Check sheet for the modelled part. Datum: model origin and axes. Units: mm. Coordinates: 2 decimals unless noted, no trailing zeros. Loops run counter-clockwise (first coordinate to the right, second up) from the corner with the lowest first, then second, coordinate; pieces in that order, holes last.
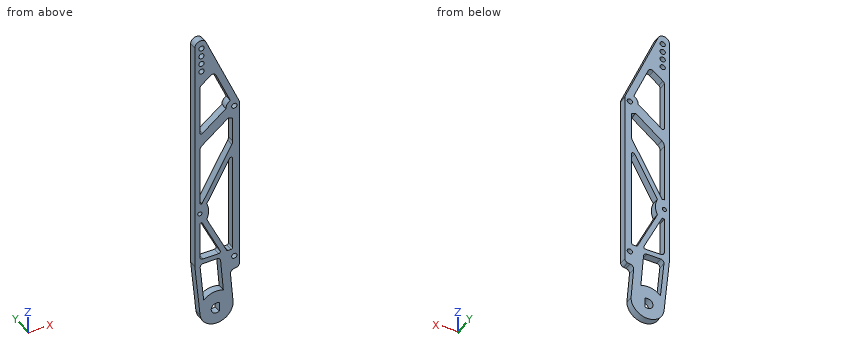
from build123d import *

# Parameters (mm, degrees)
SKETCH2_R           = 2
SKETCH2_R_2         = 1.5875
SKETCH2_R_3         = 1.999999991
BOSS_EXTRUDE1_DEPTH = 5.588


with BuildPart() as part:
    # Sketch2 → Boss-Extrude1 (new body)
    with BuildSketch(Plane(origin=(0, 0, 0), x_dir=(1, 0, 0), z_dir=(0, 1, 0))):
        with BuildLine():
            ThreePointArc((17.295902343, -30.526810701), (16.688093876, -28.878103365), (15.15555913, -28.018449791))
            Line((15.15555913, -28.018449791), (13.238676936, -27.713033224))
            ThreePointArc((13.238676936, -27.713033224), (11.241051513, -26.538356195), (10.573787778, -24.319092227))
            Line((10.573787778, -24.319092227), (12.5603, 0))
            ThreePointArc((12.5603, 0), (0.603657177, 12.545785512), (-12.502275592, 1.2059192))
            Line((-12.502275592, 1.2059192), (-16.498266045, -40.222207921))
            ThreePointArc((-16.498266045, -40.222207921), (-16.507064815, -40.344000039), (-16.51, -40.466074291))
            Line((-16.51, -40.466074291), (-16.51, -221.328861788))
            ThreePointArc((-16.51, -221.328861788), (-12.970187584, -225.680718913), (-7.988667969, -223.101301399))
            Line((-7.988667969, -223.101301399), (16.979901226, -165.677523619))
            ThreePointArc((16.979901226, -165.677523619), (17.216065593, -164.934164738), (17.295902343, -164.158289667))
            Line((17.295902343, -164.158289667), (17.295902343, -30.526810701))
        make_face()
        with Locations(Location((-11.43, -219.075, 0), (0, 0, 270))):
            Circle(SKETCH2_R, mode=Mode.SUBTRACT)
        with Locations(Location((-11.43, -212.725, 0), (0, 0, 270))):
            Circle(SKETCH2_R, mode=Mode.SUBTRACT)
        with Locations(Location((-11.43, -206.375, 0), (0, 0, 270))):
            Circle(SKETCH2_R, mode=Mode.SUBTRACT)
        with Locations(Location((-11.43, -200.025, 0), (0, 0, 270))):
            Circle(SKETCH2_R, mode=Mode.SUBTRACT)
        with BuildLine():
            ThreePointArc((7.135902343, -162.410770806), (8.023611961, -165.648962244), (10.438542905, -167.981776143))
            Line((10.438542905, -167.981776143), (-0.534170778, -193.217289931))
            ThreePointArc((-0.534170778, -193.217289931), (-2.234040931, -194.665234867), (-4.420389569, -194.211381682))
            Line((-4.420389569, -194.211381682), (-11.716886202, -188.551043102))
            ThreePointArc((-11.716886202, -188.551043102), (-12.441018517, -187.661516081), (-12.7, -186.544128716))
            Line((-12.7, -186.544128716), (-12.7, -149.615408258))
            ThreePointArc((-12.7, -149.615408258), (-11.988693683, -148.474898999), (-10.651556899, -148.611951065))
            Line((-10.651556899, -148.611951065), (7.135902343, -162.410770806))
        make_face(mode=Mode.SUBTRACT)
        with BuildLine():
            ThreePointArc((12.215902343, -152.970817152), (10.520298026, -153.359206519), (8.923603828, -154.049487576))
            Line((8.923603828, -154.049487576), (-10.733772403, -138.80005889))
            ThreePointArc((-10.733772403, -138.80005889), (-12.182037035, -137.021004847), (-12.7, -134.786230117))
            Line((-12.7, -134.786230117), (-12.7, -90.4875))
            ThreePointArc((-12.7, -90.4875), (-11.888769677, -90.445936399), (-11.086035141, -90.321680879))
            Line((-11.086035141, -90.321680879), (11.575760855, -131.079432803))
            ThreePointArc((11.575760855, -131.079432803), (12.053263487, -132.272915946), (12.215902343, -133.548047069))
            Line((12.215902343, -133.548047069), (12.215902343, -152.970817152))
        make_face(mode=Mode.SUBTRACT)
        with Locations(Location((13.485902343, -162.410770806, 0), (0, 0, 270))):
            Circle(SKETCH2_R, mode=Mode.SUBTRACT)
        with Locations(Location((-12.7, -82.55, 0), (0, 0, 270))):
            Circle(SKETCH2_R_2, mode=Mode.SUBTRACT)
        with BuildLine():
            Line((-10.16, -44.337182032), (1.663048834, -44.337182032))
            ThreePointArc((1.663048834, -44.337182032), (2.739129831, -44.932682449), (2.806066447, -46.160725831))
            Line((2.806066447, -46.160725831), (-11.055993219, -74.784618621))
            ThreePointArc((-11.055993219, -74.784618621), (-11.873503915, -74.655646925), (-12.7, -74.6125))
            Line((-12.7, -74.6125), (-12.7, -46.877182032))
            ThreePointArc((-12.7, -46.877182032), (-11.956051224, -45.081130808), (-10.16, -44.337182032))
        make_face(mode=Mode.SUBTRACT)
        with BuildLine():
            ThreePointArc((-9.903213406, -40.527182032), (-11.783508673, -39.694838236), (-12.431479451, -37.743315662))
            Line((-12.431479451, -37.743315662), (-9.755434212, -9.99962016))
            ThreePointArc((-9.755434212, -9.99962016), (-2.756273581, -13.695395429), (5.127655889, -12.99492382))
            Line((5.127655889, -12.99492382), (3.069264048, -38.19397392))
            ThreePointArc((3.069264048, -38.19397392), (2.259083254, -39.854914801), (0.537695935, -40.527182032))
            Line((0.537695935, -40.527182032), (-9.903213406, -40.527182032))
        make_face(mode=Mode.SUBTRACT)
        with BuildLine():
            ThreePointArc((2.05, -3.492849839), (-4.05, 0), (2.05, 3.492849839))
            Line((2.05, 3.492849839), (2.05, -3.492849839))
        make_face(mode=Mode.SUBTRACT)
        with BuildLine():
            ThreePointArc((-7.44734835, -89.025591197), (-5.976040897, -82.55), (-7.44734835, -76.074408803))
            Line((-7.44734835, -76.074408803), (7.575478058, -45.053638233))
            ThreePointArc((7.575478058, -45.053638233), (8.043996088, -44.531101035), (8.718495671, -44.337182032))
            Line((8.718495671, -44.337182032), (10.945902343, -44.337182032))
            ThreePointArc((10.945902343, -44.337182032), (11.843927955, -44.70915642), (12.215902343, -45.607182032))
            Line((12.215902343, -45.607182032), (12.215902343, -119.492817968))
            ThreePointArc((12.215902343, -119.492817968), (11.264685124, -120.722158254), (9.835937715, -120.109971535))
            Line((9.835937715, -120.109971535), (-7.44734835, -89.025591197))
        make_face(mode=Mode.SUBTRACT)
        with Locations(Location((13.485902343, -38.1, 0), (0, 0, 270))):
            Circle(SKETCH2_R_3, mode=Mode.SUBTRACT)
    extrude(amount=BOSS_EXTRUDE1_DEPTH)


solid = part.part
(1) Gauge pin test, flat ends, axial feed: P1, Ø1, axis at x = -4.5, y = 4, coming from the +Z side; P2, Ø3, axis at x = -4, y = 3, coming from the +Z side; P3, Ø1, axis at x = 8, y = 1, coming from the -Z side. Record the tip position at first contact, or that the pin passes through.
(2) Scan lines: line 1 along X through (y, z) = (2.55, 118); line 2 along Z through (x, y) = (-8.5, 5); line 3 along X through (y, z) = (0.8, 107.5). Record each from-to range of solid material in increasing order.
(3) Section check A-A, the plane z = 60. Enter the section's corners in (x, y), plus the area to 3 significant figures.
Determined:
1. P1: stops at z = 216.23
1. P2: stops at z = 217.38
1. P3: stops at z = -10.08
2. line 1: x = -16.51 to -12.7, 4.3 to 8.66, 12.22 to 17.3
2. line 2: z = -9.25 to 11.09, 40.53 to 44.34, 69.51 to 94.97, 140.53 to 150.28, 191.05 to 223.98
2. line 3: x = -16.51 to -12.7, -1.53 to 2.82, 12.22 to 17.3
3. outline: (-16.51, 0) - (-12.7, 0) - (-12.7, 5.59) - (-16.51, 5.59) - close; (-3.9, 0) - (0.34, 0) - (0.34, 5.59) - (-3.9, 5.59) - close; (12.22, 0) - (17.3, 0) - (17.3, 5.59) - (12.22, 5.59) - close
3. area: 73.3 mm2
